```python
from build123d import *

# Parameters (mm, degrees)
BOSS_EXTRUDE1_DEPTH      = 75
BOSS_EXTRUDE1_DEPTH_BACK = 75
SKETCH1_W                = 100
SKETCH1_H                = 100
SKETCH2_W                = 35
SKETCH2_H                = 100
CUT_EXTRUDE1_DEPTH       = 80
CUT_EXTRUDE2_DEPTH       = 136
SKETCH5_W                = 60
SKETCH5_H                = 60
CUT_EXTRUDE3_DEPTH       = 80
SKETCH6_W                = 60
SKETCH6_H                = 10
CUT_EXTRUDE5_DEPTH       = 166.831239518
CUT_EXTRUDE6_DEPTH       = 121.519707932
HOLE1_D                  = 30


with BuildPart() as part:
    # Sketch1 → Boss-Extrude1 (new, two sides: drawn at the far end of the back side and taken through both)
    with BuildSketch(Plane(origin=(0, 0, 0), x_dir=(0, 0, -1), z_dir=(1, 0, 0)).offset(-BOSS_EXTRUDE1_DEPTH_BACK)):
        Rectangle(SKETCH1_W, SKETCH1_H)
    extrude(amount=BOSS_EXTRUDE1_DEPTH + BOSS_EXTRUDE1_DEPTH_BACK)

    # Sketch2 → Cut-Extrude1 (cut)
    with BuildSketch(Plane(origin=(0, 50, 0), x_dir=(1, 0, 0), z_dir=(0, 1, 0))):
        with Locations((57.5, 0)):
            Rectangle(SKETCH2_W, SKETCH2_H)
        with Locations((-57.5, 0)):
            Rectangle(SKETCH2_W, SKETCH2_H)
    extrude(amount=-CUT_EXTRUDE1_DEPTH, mode=Mode.SUBTRACT)

    # Sketch3 → Cut-Extrude2 (cut, through all)
    with BuildSketch(Plane(origin=(40, 0, 0), x_dir=(0, 0, -1), z_dir=(1, 0, 0))):
        Polygon((30, 50), (-50, -10), (-50, 50), align=None)
    extrude(amount=-CUT_EXTRUDE2_DEPTH, mode=Mode.SUBTRACT)

    # Sketch5 → Cut-Extrude3 (cut)
    with BuildSketch(Plane.XY.offset(50)):
        with Locations((0, 10)):
            Rectangle(SKETCH5_W, SKETCH5_H)
    extrude(amount=-CUT_EXTRUDE3_DEPTH, mode=Mode.SUBTRACT)

    # Sketch6 → Cut-Extrude5 (cut, through all)
    with BuildSketch(Plane(origin=(75, 0, 0), x_dir=(0, 0, -1), z_dir=(1, 0, 0))):
        with Locations((0, -45)):
            Rectangle(SKETCH6_W, SKETCH6_H)
    extrude(amount=-CUT_EXTRUDE5_DEPTH, mode=Mode.SUBTRACT)

    # Sketch7 → Cut-Extrude6 (cut, through all)
    with BuildSketch(Plane(origin=(0, -30, 0), x_dir=(1, 0, 0), z_dir=(0, 1, 0))):
        with BuildLine():
            Line((59.99999901, 3.75), (75, 3.75))
            Line((75, 3.75), (75, -3.75))
            Line((75, -3.75), (60, -3.75))
            ThreePointArc((60, -3.75), (56.25, -4.95e-07), (59.99999901, 3.75))
        make_face()
    cut_extrude6 = extrude(amount=-CUT_EXTRUDE6_DEPTH, mode=Mode.SUBTRACT)

    # Mirror1: Cut-Extrude6 across plane
    add(cut_extrude6.mirror(Plane(origin=(0, 0, 0), x_dir=(0, 0, 1), z_dir=(1, 0, 0))), mode=Mode.SUBTRACT)

    # Hole1 (through all)
    with Locations(Plane.XY.offset(-30)):
        with Locations((0, 10)):
            Hole(HOLE1_D / 2)


solid = part.part
```
For this review, take the finished solid that the model builds, in its own axes (mm). A direction names the side the tool comes from. Round coordinates to 2 decimals unless told otherwise and drop trailing zeros. Write each loop counter-clockwise with the first axis right and the second up, starting at its lowest first coordinate (ties: lowest second). Pieces come first, ordered by that corner, then holes. Notation, with made-up numbers: (18, 68) - (45, 68) arc R21 ccw to (45, 82) - close; hole circle Ø6 at (64, 82.25). An arc over 180 degrees is marked (long way). Answer as CSV lines item,"result". Start each with the question number.
(1) For line 1 (X direction, y = 10.5, z = -26); line 2 (Y direction, x = 0, z = -44.75); line 3 (X direction, y = -28, z = 18.5), list the stretches that pass through material, from the lowest coordinate up.
(2) Machinability: for faces 5 (the flat face through (53, -30, -1)), 6 (the flat face through (1, -45, 30)), 7 (the flat face through (0, 40, -23)), which of the approach directions +Z, -Z, +X, -X, +Y, -Y give a long, thin tool a straight path to every point of the face, cutting with its end or side? Answer none if there is none.
(3) Add section C-C, the plane y = 35. State the section outline as (x, z) points, plus the area to 3 significant figures.
(4) Add section B-B, the plane z = -23. State the section outline as (x, y) points.
(5) Add section A-A, the plane x = 0. State the section outline as (y, z) points.
(6) For pin 1 (10.5 mm diameter, centred on x = 65.5, z = -21.5, fed in from +Y); pin 2 (8 mm diameter, centred on y = 10.5, z = 6.5, fed in from -X); pin 3 (24 mm diameter, centred on y = 17.5, z = -20.5, fed in from +X), all flat-tipped, find the tip position at first contact; note any pin that passes through.
(7) Add section D-D, the plane y = 1. State the section outline as (x, z) points.
(8) Mouldability with a two-part tool opening along X and no side actions: class faces 1 (the flat face through (40, 2, -10)), 2 (the flat face through (-1, -50, 40)), 3 (the flat face through (-75, -38, -32)), 4 (the flat face through (-7, 24, -30)) as +X half, -X half, draft (parallel to the pull), parting line (faces both ways), or undercut.
From the geometry:
1,line 1,"x = -40 to -30, 30 to 40"
1,line 2,"y = -50 to -5, 25 to 50"
1,line 3,"x = -40 to 40"
2,face 5,"+Z, -Z, +X, +Y"
2,face 6,"+X, -X, -Y"
2,face 7,"+Z"
3,outline,"(-40, -50) - (40, -50) - (40, -10) - (30, -10) - (30, -30) - (-30, -30) - (-30, -10) - (-40, -10) - close"
3,area,"2,000 mm²"
4,outline,"(-75, -40) - (75, -40) - (75, -30) - (40, -30) - (40, 44.75) - (-40, 44.75) - (-40, -30) - (-75, -30) - close; hole (-30, -20) - (30, -20) - (30, 40) - (-30, 40) - close"
5,outline,"(-50, -50) - (-5, -50) - (-5, -30) - (-20, -30) - (-20, 50) - (-50, 50) - (-50, 30) - (-40, 30) - (-40, -30) - (-50, -30) - close; (25, -50) - (50, -50) - (50, -30) - (40, -16.67) - (40, -30) - (25, -30) - close"
6,pin 1,"stops at y = -30"
6,pin 2,"stops at x = -40"
6,pin 3,"stops at x = 40"
7,outline,"(-40, -50) - (-12, -50) - (-12, -30) - (-30, -30) - (-30, 35.33) - (-40, 35.33) - close; (12, -50) - (40, -50) - (40, 35.33) - (30, 35.33) - (30, -30) - (12, -30) - close"
8,face 1,"+X half"
8,face 2,"draft"
8,face 3,"-X half"
8,face 4,"undercut"
